Part print with two shaded views. Sizes in mm from the minimum x, y, z corner. A direction names the side the tool comes from. Give positions to 0.01 mm unless a question says otherwise; leave off trailing zeros. Loops run counter-clockwise (first coordinate to the right, second up) from the corner with the lowest first, then second, coordinate; pieces in that order, holes last. Notation, with made-up numbers: (26.5, -17.5) -> (73.5, -17.5) arc R30 cw to (73.5, 8.5) -> close; hole circle Ø9 at (-5.5, 9.5). An arc over 180 degrees is marked (long way). One line per question, with ' | ' between items.
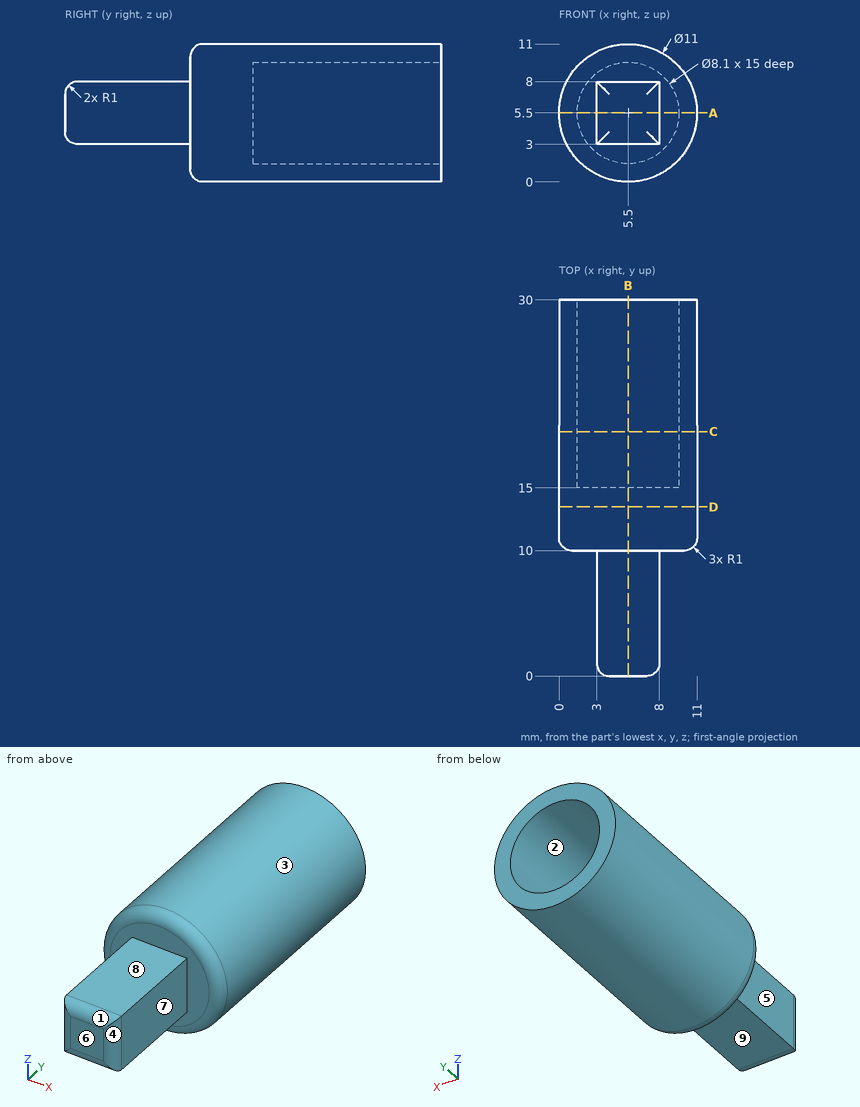
1) Pull direction Z, two halves, no side cores. Call the marked faces 1, 2, 3 and 4: pulls with the +Z half, pulls with the -Z half, needs draft (parallel to the pull), parting line crosses it, or undercut.
Found:
face 1: pulls with the +Z half | face 2: undercut | face 3: parting line crosses it | face 4: needs draft
2) Saw through at B-B (x = 5.5). Give the cut face in (y, z).
Found:
outline: (0, 4) arc R1 ccw to (1, 3) -> (10, 3) -> (10, 1) arc R1 ccw to (11, 0) -> (30, 0) -> (30, 1.45) -> (15, 1.45) -> (15, 9.55) -> (30, 9.55) -> (30, 11) -> (11, 11) arc R1 ccw to (10, 10) -> (10, 8) -> (1, 8) arc R1 ccw to (0, 7) -> close
3) Tool access for the marked faces 5, 6, 7, 8 and 9: list every direction of +Z, -Z, +X, -X, +Y, -Y with a clear straight run to the whole face (end or side of a thin tool).
Found:
face 5: +Z, -Z, -X, -Y | face 6: +Z, -Z, +X, -X, -Y | face 7: +Z, -Z, +X, -Y | face 8: +Z, +X, -X, -Y | face 9: -Z, +X, -X, -Y
4) Saw through at C-C (y = 19.5). Give the cut face in (x, z), and give its area (3 significant figures).
Found:
outline: circle Ø11 at (5.5, 5.5); hole circle Ø8.1 at (5.5, 5.5) | area: 43.5 mm2
5) Saw through at A-A (z = 5.5). Give the cut face in (x, y).
Found:
outline: (0, 11) arc R1 ccw to (1, 10) -> (3, 10) -> (3, 1) arc R1 ccw to (4, 0) -> (7, 0) arc R1 ccw to (8, 1) -> (8, 10) -> (10, 10) arc R1 ccw to (11, 11) -> (11, 30) -> (9.55, 30) -> (9.55, 15) -> (1.45, 15) -> (1.45, 30) -> (0, 30) -> close
6) Pin check, flat tips, straight feed: P1, Ø2, axis at x = 9.5, y = 10, coming from the -Z side; P2, Ø5.5, axis at y = 6.5, z = 5.5, coming from the -X side; P3, Ø2.5, axis at y = 7.5, z = 4.5, coming from the +X side. Stop position of each tip, or through.
Found:
P1: z = 1.13 | P2: x = 3 | P3: x = 8
7) Drill centre lines: line 1 (Z direction, x = 5.5, y = 25.5); line 2 (Y direction, x = 6.5, z = 6). Where is each one in solid material? Low to high.
Found:
line 1: 0 to 1.45, 9.55 to 11 | line 2: 0 to 15
8) Saw through at D-D (y = 13.5). Give the cut face in (x, z).
Found:
outline: circle Ø11 at (5.5, 5.5)
